from build123d import *

# Parameters (mm, degrees)
F0_R     = 4.7625
F0_R_2   = 23.8125
F1_DEPTH = 6.35


# Not quite as in the source:
# - the program builds the solid bodies; features that only make, move or delete a surface that nothing else refers to are left out


with BuildPart() as f1:
    # F0 (on Front) → F1 (new body)
    with BuildSketch(Plane.XZ):
        Polygon((-25.6632194655, 44.45), (-51.326438931, 0), (-25.6632194655, -44.45), (25.6632194655, -44.45), (51.326438931, 0), (25.6632194655, 44.45), align=None)
        with Locations((-28.5741617877, -16.4973)):
            Circle(F0_R, mode=Mode.SUBTRACT)
        with Locations((28.5741617877, -16.4973)):
            Circle(F0_R, mode=Mode.SUBTRACT)
        Circle(F0_R_2, mode=Mode.SUBTRACT)
        with Locations((0, 32.9946)):
            Circle(F0_R, mode=Mode.SUBTRACT)
    extrude(amount=-F1_DEPTH)


solid = f1.part
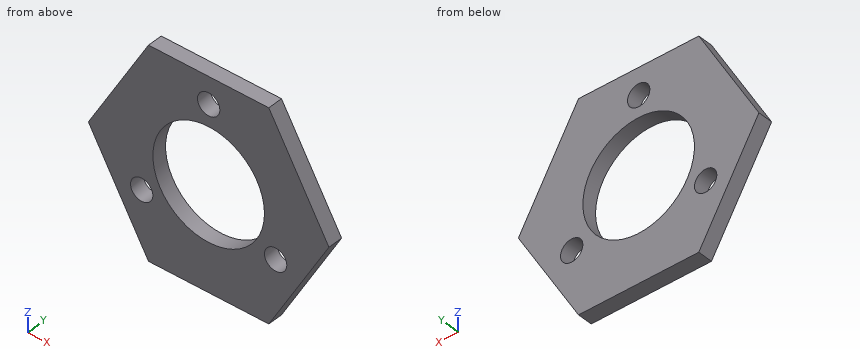
Check sheet for the modelled part. Datum: model origin and axes. Units: mm. Give positions to 0.01 mm unless a question says otherwise; leave off trailing zeros. Loops run counter-clockwise (first coordinate to the right, second up) from the corner with the lowest first, then second, coordinate; pieces in that order, holes last. Notation, with made-up numbers: M 58,4 L 94,4 A14 cw 94,15 Z; hole C 44.5,-39.5 d10. An arc over 180 degrees is marked long. Answer as a JSON object with one key per item and string values. Group by question number.
Q1. Cross-section at C-C on z = 3. Record the cut outline in (x, y), then the cut area to 3 significant figures.
Q2. Go/stop test with flat-tipped pins: P1, Ø1, axis at x = 34, y = 4, coming from the -Z side; P2, Ø8.5, axis at x = 28.57, z = -16.5, coming from the +Y side. Record where each tip stops, or that it passes through.
Q3. Cross-section at A-A on x = 0. Record the cut outline in (y, z), then the cut area to 3 significant figures.
Q4. Cross-section at B-B on x = -21. Record the cut outline in (y, z), then the cut area to 3 significant figures.
Q5. Cross-section at D-D on y = 5.25. Give the number of separate pieces and of enclosed holes in the cut face, then the cut area to 3 significant figures.
Q6. Material ranges on line 1 along Z through (x, y) = (0, 5); line 2 along X through (y, z) = (1, -14.5); line 3 along X through (y, z) = (2.25, 5), recorded low to high. Write a range as [from, to].
Evaluation:
{
 "1": {"outline": "M -49.59,0 L -23.62,0 L -23.62,6.35 L -49.59,6.35 Z; M 23.62,0 L 49.59,0 L 49.59,6.35 L 23.62,6.35 Z", "area": "330 mm2"},
 "2": {"P1": "stops at z = -30.88", "P2": "passes through"},
 "3": {"outline": "M 0,-44.45 L 6.35,-44.45 L 6.35,-23.81 L 0,-23.81 Z; M 0,23.81 L 6.35,23.81 L 6.35,28.23 L 0,28.23 Z; M 0,37.76 L 6.35,37.76 L 6.35,44.45 L 0,44.45 Z", "area": "202 mm2"},
 "4": {"outline": "M 0,-44.45 L 6.35,-44.45 L 6.35,-11.23 L 0,-11.23 Z; M 0,11.23 L 6.35,11.23 L 6.35,44.45 L 0,44.45 Z", "area": "422 mm2"},
 "5": {"separate pieces": "1", "enclosed holes": "4", "area": "4,850 mm2"},
 "6": {"line 1": "z = [-44.45, -23.81], [23.81, 28.23], [37.76, 44.45]", "line 2": "x = [-42.95, -32.9], [-24.25, -18.89], [18.89, 24.25], [32.9, 42.95]", "line 3": "x = [-48.44, -23.28], [23.28, 48.44]"}
}
